Here's the drawing with two shaded views (mm, measured from the low corner). I have some questions. Coordinates: 2 decimals unless noted, no trailing zeros. Loops run counter-clockwise (first coordinate to the right, second up) from the corner with the lowest first, then second, coordinate; pieces in that order, holes last. Notation, with made-up numbers: (-15, 40.25) - (17, 40.25) arc R31 cw to (17, 65.25) - close; hole circle Ø7 at (62.25, 2). An arc over 180 degrees is marked (long way). Use a Markdown table: item, result.
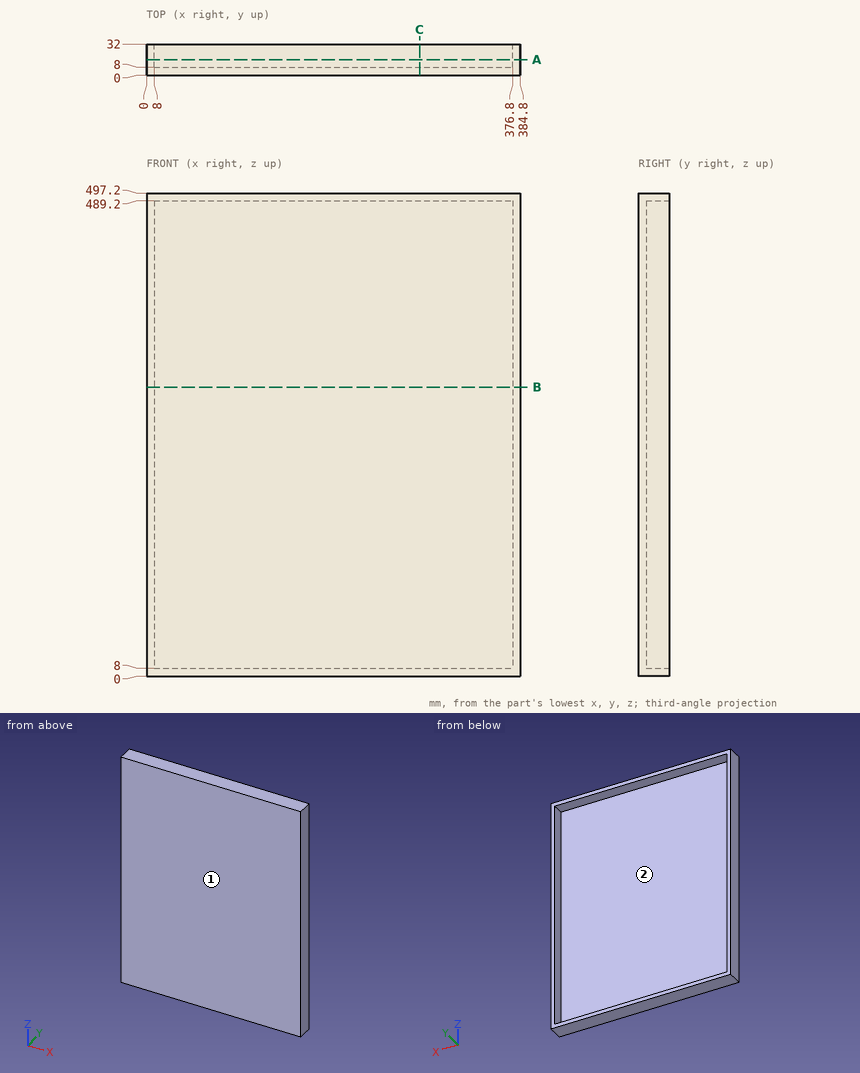
Q1. Please list where these lines run through material, in increasing order: L1, parallel to Z at x = 180.5, y = 24; L2, parallel to X at y = 17, z = 299.5; L3, parallel to Y at x = 249, z = 287. Write a range as from..to.
Check values:
| item | result |
|---|---|
| L1 | 0..8, 489.2..497.2 |
| L2 | 0..8, 376.8..384.8 |
| L3 | 0..8 |
Q2. I want a section at A-A, the plane y = 16. Write out the boundary of the cut face in (x, z), then the cut area to 3 significant figures.
Check values:
| item | result |
|---|---|
| outline | (0, 0) - (384.8, 0) - (384.8, 497.2) - (0, 497.2) - close; hole (8, 8) - (376.8, 8) - (376.8, 489.2) - (8, 489.2) - close |
| area | 13,900 mm^2 |
Q3. I want a section at B-B, the plane z = 297.5. Write out the boundary of the cut face in (x, y), then the cut area to 3 significant figures.
Check values:
| item | result |
|---|---|
| outline | (0, 0) - (384.8, 0) - (384.8, 32) - (376.8, 32) - (376.8, 8) - (8, 8) - (8, 32) - (0, 32) - close |
| area | 3,460 mm^2 |
Q4. Will this pin go through, and if not, where does the flat tip stop? P1, Ø6, axis at x = 154, z = 100.5, coming from the +Y side.
Check values:
| item | result |
|---|---|
| P1 | y = 8 |
Q5. I want a section at C-C, the plane x = 281. Write out the boundary of the cut face in (y, z), then the cut area to 3 significant figures.
Check values:
| item | result |
|---|---|
| outline | (0, 0) - (32, 0) - (32, 8) - (8, 8) - (8, 489.2) - (32, 489.2) - (32, 497.2) - (0, 497.2) - close |
| area | 4,360 mm^2 |
Q6. If we mould it in two halves opening along Z, with no side actions, what happens to the marked faces 1 and 2? For each: pulls with the +Z half, pulls with the -Z half, needs draft (parallel to the pull), parting line crosses it, or undercut.
Check values:
| item | result |
|---|---|
| face 1 | needs draft |
| face 2 | undercut |
